Geometry check sheet. Reference: the model listing, model coordinates, mm. A direction names the side the tool comes from. Give positions to 0.01 mm unless a question says otherwise; leave off trailing zeros. Order: outer loops, then holes, each group sorted by start corner. A loop starts at its lowest first (then second) coordinate and runs counter-clockwise, first axis right, second up.
```python
from build123d import *

# Parameters (mm, degrees)
SKETCH1_W           = 125
SKETCH1_H           = 94
BOSS_EXTRUDE2_DEPTH = 9
SKETCH2_W           = 16
SKETCH2_H           = 23
BOSS_EXTRUDE4_DEPTH = 100
SKETCH4_W           = 12
SKETCH4_H           = 17
CUT_EXTRUDE1_DEPTH  = 96.5
SKETCH5_R           = 5
CUT_EXTRUDE2_DEPTH  = 100
CUT_EXTRUDE3_START  = 8.777087
SKETCH6_W           = 19
SKETCH6_H           = 4
CUT_EXTRUDE3_DEPTH  = 100
SKETCH7_R           = 2
SKETCH7_R_2         = 2.002973214
SKETCH7_R_3         = 2.108586534
SKETCH7_R_4         = 2.000351704
CUT_EXTRUDE4_DEPTH  = 100
SKETCH8_W           = 62
SKETCH8_H           = 62
BOSS_EXTRUDE5_DEPTH = 9


with BuildPart() as part:
    # Sketch1 → Boss-Extrude2 (new body)
    with BuildSketch(Plane(origin=(0, 0, 0), x_dir=(1, 0, 0), z_dir=(0, 1, 0))):
        with Locations((0.777087034, -16.027531083)):
            Rectangle(SKETCH1_W, SKETCH1_H)
    extrude(amount=BOSS_EXTRUDE2_DEPTH)

    # Sketch2 → Boss-Extrude4 (add)
    with BuildSketch(Plane(origin=(0, 0, 0), x_dir=(1, 0, 0), z_dir=(0, 1, 0))):
        with Locations((0.777087034, -16.027531083)):
            Rectangle(SKETCH2_W, SKETCH2_H)
    extrude(amount=BOSS_EXTRUDE4_DEPTH)

    # Sketch4 → Cut-Extrude1 (cut)
    with BuildSketch(Plane(origin=(0, 0, 0), x_dir=(1, 0, 0), z_dir=(0, 1, 0))):
        with Locations((0.777087034, -16.027531083)):
            Rectangle(SKETCH4_W, SKETCH4_H)
    extrude(amount=CUT_EXTRUDE1_DEPTH, mode=Mode.SUBTRACT)

    # Sketch5 → Cut-Extrude2 (cut)
    with BuildSketch(Plane(origin=(0, 100, 0), x_dir=(1, 0, 0), z_dir=(0, 1, 0))):
        with Locations(Location((0.905359977, -15.45030284, 0), (0, 0, 270))):
            Circle(SKETCH5_R)
    extrude(amount=-CUT_EXTRUDE2_DEPTH, mode=Mode.SUBTRACT)

    # Sketch6 → Cut-Extrude3 (cut)
    with BuildSketch(Plane(origin=(0, 0, 0), x_dir=(0, 0, -1), z_dir=(1, 0, 0)).offset(CUT_EXTRUDE3_START)):
        with Locations((-15.823546724, 95)):
            Rectangle(SKETCH6_W, SKETCH6_H)
    extrude(amount=-CUT_EXTRUDE3_DEPTH, mode=Mode.SUBTRACT)

    # Sketch7 → Cut-Extrude4 (cut)
    with BuildSketch(Plane(origin=(0, 0, 0), x_dir=(1, 0, 0), z_dir=(0, 1, 0))):
        with Locations(Location((-54.512912966, 25.852468917, 0), (0, 0, 270))):
            Circle(SKETCH7_R)
        with Locations(Location((57.335663159, 25.288094206, 0), (0, 0, 270))):
            Circle(SKETCH7_R_2)
        with Locations(Location((57.809152834, -57.571905794, 0), (0, 0, 270))):
            Circle(SKETCH7_R_3)
        with Locations(Location((-54.169424944, -57.007531083, 0), (0, 0, 270))):
            Circle(SKETCH7_R_4)
    extrude(amount=CUT_EXTRUDE4_DEPTH, mode=Mode.SUBTRACT)

    # Sketch8 → Boss-Extrude5 (add)
    with BuildSketch(Plane(origin=(0, 0, 0), x_dir=(1, 0, 0), z_dir=(0, 1, 0))):
        with Locations((-92.722912966, -16.947525928)):
            Rectangle(SKETCH8_W, SKETCH8_H)
    extrude(amount=BOSS_EXTRUDE5_DEPTH)


solid = part.part
```
Q1. Gauge pin test, flat ends, axial feed: P1, Ø7, axis at x = -101.5, y = 3, coming from the +Z side; P2, Ø4.5, axis at y = 5.5, z = 58, coming from the -X side; P3, Ø3.5, axis at x = -1, y = 55, coming from the +Z side. Record the tip position at first contact, or that the pin passes through.
Q2. Cross-section at B-B, the plane z = 13. Record the boundary of the cut face in (x, y), and give its area (3 significant figures).
Q3. Cross-section at A-A, the plane y = 88.5. Record the boundary of the cut face in (x, z), and give its area (3 significant figures).
Q4. Cross-section at D-D, the plane y = 6. Record the boundary of the cut face in (x, z).
Q5. Thickness scan on L1, parallel to Z at x = 3, y = 24; L2, parallel to X at y = 11, z = 11.5; L3, parallel to Y at x = 28, z = -10. Record the ranges inside material, lowest first.
Q6. Cross-section at C-C, the plane x = -92.5. Record the boundary of the cut face in (y, z), and give its area (3 significant figures).
Q7. Release check for a two-part mould opening along Z. For faces 1 (the face through (-93, 4, -14.052)), 2 (the face through (55.38, 4.44, -25.72)), 3 (the face through (56.526, 4.437, 55.899)), 4 (the face through (-93, 4, 47.948)) record: pulls with the +Z half, pulls with the -Z half, needs draft (parallel to the pull), parting line crosses it, or undercut.
Q8. Access from +Z, -Z, +X, -X, +Y, -Y to the whole of each face (thin tool, end or side, straight path). Record for faces 5 (the face through (1, 95, 6.324)), 6 (the face through (-61.723, 4, -22)), 7 (the face through (1, 46, 7.528)), 8 (the face through (1, 54, 4.528)).
Answers follow:
1. P1: stops at z = 47.95
1. P2: stops at x = -61.72
1. P3: stops at z = 27.53
2. outline: (-123.72, 0) - (-5.22, 0) - (-5.22, 93) - (-7.22, 93) - (-7.22, 9) - (-123.72, 9) - close; (-7.22, 97) - (-3.45, 97) - (-3.45, 100) - (-7.22, 100) - close; (5.26, 97) - (8.78, 97) - (8.78, 100) - (5.26, 100) - close; (6.78, 0) - (63.28, 0) - (63.28, 9) - (8.78, 9) - (8.78, 93) - (6.78, 93) - close
2. area: 1,930 mm2
3. outline: (-7.22, 4.53) - (8.78, 4.53) - (8.78, 27.53) - (-7.22, 27.53) - close; hole (-5.22, 7.53) - (6.78, 7.53) - (6.78, 24.53) - (-5.22, 24.53) - close
3. area: 164 mm2
4. outline: (-123.72, -14.05) - (-61.72, -14.05) - (-61.72, -30.97) - (63.28, -30.97) - (63.28, 63.03) - (-61.72, 63.03) - (-61.72, 47.95) - (-123.72, 47.95) - close; hole circle Ø4 at (-54.51, -25.85); hole circle Ø4 at (-54.17, 57.01); hole (-5.22, 7.53) - (6.78, 7.53) - (6.78, 24.53) - (-5.22, 24.53) - close; hole circle Ø4.01 at (57.34, -25.29); hole circle Ø4.22 at (57.81, 57.57)
5. L1: z = 4.53 to 7.53, 24.53 to 27.53
5. L2: x = -7.22 to -5.22, 6.78 to 8.78
5. L3: y = 0 to 9
6. outline: (0, -14.05) - (9, -14.05) - (9, 47.95) - (0, 47.95) - close
6. area: 558 mm2
7. face 1: pulls with the -Z half
7. face 2: undercut
7. face 3: undercut
7. face 4: pulls with the +Z half
8. face 5: +X, -X
8. face 6: -Z, -X, +Y, -Y
8. face 7: -Y
8. face 8: -Z, +X, -X, +Y
